Could you check a few things on this model? Use its own coordinates, in mm. A direction names the side the tool comes from. Coordinates: 2 decimals unless noted, no trailing zeros. Write each loop counter-clockwise with the first axis right and the second up, starting at its lowest first coordinate (ties: lowest second). Pieces come first, ordered by that corner, then holes. Notation, with made-up numbers: (33.5, 53.25) - (53.5, 53.25) arc R21 ccw to (53.5, 86.25) - close; hole circle Ø3 at (31, 43.25). An arc over 180 degrees is marked (long way). Answer as a JSON object with one key per item and string values. Group by question number.
1) We'd pull the mould along X, two halves only. Please class faces 1 (the cylindrical face through (14.447, -6.535, -0.045)), 2 (the flat face through (19.8, -5, 0)), 3 (the flat face through (7, 1, -1.15)): released by +X, released by -X, zero draft, split by the parting line, or undercut.
2) If we section it at C-C (x = 14.6): Write out the boundary of the cut face in (y, z) (3 decimals).
3) If we section it at A-A (y = -7.7): Write out the boundary of the cut face in (x, z) (3 decimals), plus the area to 3 significant figures.
4) Will these pins go through, and if not, where does the flat tip stop? pin 1 Ø1.5 at (x, z) = (11, 1.5) entering from -Y; pin 2 Ø3 at (x, z) = (14.5, 0) entering from +Y; pin 3 Ø0.5 at (y, z) = (0.5, -0.5) entering from -X.
5) On a 3-axis mill with a long thin cutter (end or side, diameter ignored), from which of +Z, -Z, +X, -X, +Y, -Y can I reach the whole of each face in a straight line? I mean faces 4 (the flat face through (7, 1, 1.15)), 5 (the flat face through (9.96, 3.305, 0.016)), 6 (the flat face through (8.1, 0.6, 0)), 7 (the flat face through (6.1, 0.6, 0)), 8 (the flat face through (10, -5, -3.2)). Say none if no direction works.
6) If we section it at B-B (z = 2.5): Write out the boundary of the cut face in (x, y) (3 decimals), plus the area to 3 significant figures.
7) If we section it at D-D (x = 8.5): Write out the boundary of the cut face in (y, z).
8) Please list where these lines run through material, in increasing order: line 1 along Y through (x, z) = (5.1, 1.5) (3 decimals); line 2 along Y through (x, z) = (14.6, 1.75) (3 decimals); line 3 along Y through (x, z) = (4.75, 0).
```python
from build123d import *

# Parameters (mm, degrees)
SKETCH_1_R       = 1.175
EXTRUDE_1_DEPTH  = 3.2
EXTRUDE_2_DEPTH  = 1.15
EXTRUDE_10_DEPTH = 1.15
SKETCH_5_W       = 0.3
SKETCH_5_H       = 3
EXTRUDE_12_DEPTH = 0.25


with BuildPart() as part:
    # 草图1 → 凸台-拉伸1 (new, symmetric)
    with BuildSketch(Plane.XY):
        with BuildLine():
            Line((0.5, 0), (9.1, 0))
            Line((9.1, 0), (9.8, -0.7))
            Line((9.8, -0.7), (19.3, -0.7))
            ThreePointArc((19.3, -0.7), (19.653553391, -0.846446609), (19.8, -1.2))
            Line((19.8, -1.2), (19.8, -9.7))
            ThreePointArc((19.8, -9.7), (19.653553391, -10.053553391), (19.3, -10.2))
            Line((19.3, -10.2), (0.5, -10.2))
            ThreePointArc((0.5, -10.2), (0.146446609, -10.053553391), (0, -9.7))
            Line((0, -9.7), (0, -0.5))
            ThreePointArc((0, -0.5), (0.146446609, -0.146446609), (0.5, 0))
        make_face()
        with Locations((5.1, -7.7)):
            Circle(SKETCH_1_R, mode=Mode.SUBTRACT)
        with Locations((14.6, -7.7)):
            Circle(SKETCH_1_R, mode=Mode.SUBTRACT)
    extrude(amount=EXTRUDE_1_DEPTH, both=True)

    # 草图2 → 凸台-拉伸2 (add, symmetric)
    with BuildSketch(Plane.XY):
        with BuildLine():
            Line((6.1, 1.118033989), (6.1, 0))
            Line((6.1, 0), (8.1, 0))
            Line((8.1, 0), (8.1, 1.118033989))
            ThreePointArc((8.1, 1.118033989), (7.1, 1.5), (6.1, 1.118033989))
        make_face()
    extrude(amount=EXTRUDE_2_DEPTH, both=True)

    # 草图4 → 凸台-拉伸10 (add, symmetric)
    with BuildSketch(Plane.XY):
        Polygon((2.85, 0), (3.15, 0), (3.15, 0.4), (16.98060531, 5.648457972), (16.874167088, 5.928941314), (2.85, 0.60703024), align=None)
    extrude(amount=EXTRUDE_10_DEPTH, both=True)

    # 草图5 → 凸台-拉伸12 (add, symmetric)
    with BuildSketch(Plane.XY):
        with Locations((1.6, -11.7)):
            Rectangle(SKETCH_5_W, SKETCH_5_H)
        with Locations((10.4, -11.7)):
            Rectangle(SKETCH_5_W, SKETCH_5_H)
        with Locations((17.7, -11.7)):
            Rectangle(SKETCH_5_W, SKETCH_5_H)
    extrude(amount=EXTRUDE_12_DEPTH, both=True)


solid = part.part
```
Here are the results:
{
 "1": {"face 1": "undercut", "face 2": "released by +X", "face 3": "zero draft"},
 "2": {"outline": "(-10.2, -3.2) - (-8.875, -3.2) - (-8.875, 3.2) - (-10.2, 3.2) - close; (-6.525, -3.2) - (-0.7, -3.2) - (-0.7, 3.2) - (-6.525, 3.2) - close; (4.745, -1.15) - (5.066, -1.15) - (5.066, 1.15) - (4.745, 1.15) - close"},
 "3": {"outline": "(0, -3.2) - (3.925, -3.2) - (3.925, 3.2) - (0, 3.2) - close; (6.275, -3.2) - (13.425, -3.2) - (13.425, 3.2) - (6.275, 3.2) - close; (15.775, -3.2) - (19.8, -3.2) - (19.8, 3.2) - (15.775, 3.2) - close", "area": "96.6 mm²"},
 "4": {"pin 1": "stops at y = -10.2", "pin 2": "stops at y = 5.6", "pin 3": "stops at x = 2.85"},
 "5": {"face 4": "+Z, +X, -X, +Y", "face 5": "+Z, -Z, -X, +Y", "face 6": "+Z, -Z, +X", "face 7": "+Z, -Z", "face 8": "-Z, +X, -X, +Y, -Y"},
 "6": {"outline": "(0, -9.7) arc R0.5 ccw to (0.5, -10.2) - (19.3, -10.2) arc R0.5 ccw to (19.8, -9.7) - (19.8, -1.2) arc R0.5 ccw to (19.3, -0.7) - (9.8, -0.7) - (9.1, 0) - (0.5, 0) arc R0.5 ccw to (0, -0.5) - close; hole circle Ø2.35 at (5.1, -7.7); hole circle Ø2.35 at (14.6, -7.7)", "area": "186 mm²"},
 "7": {"outline": "(-10.2, -3.2) - (0, -3.2) - (0, 3.2) - (-10.2, 3.2) - close; (2.43, -1.15) - (2.75, -1.15) - (2.75, 1.15) - (2.43, 1.15) - close"},
 "8": {"line 1": "y = -10.2 to -8.875, -6.525 to 0", "line 2": "y = -10.2 to -8.875, -6.525 to -0.7", "line 3": "y = -10.2 to -8.82, -6.58 to 0, 1.01 to 1.33"}
}
